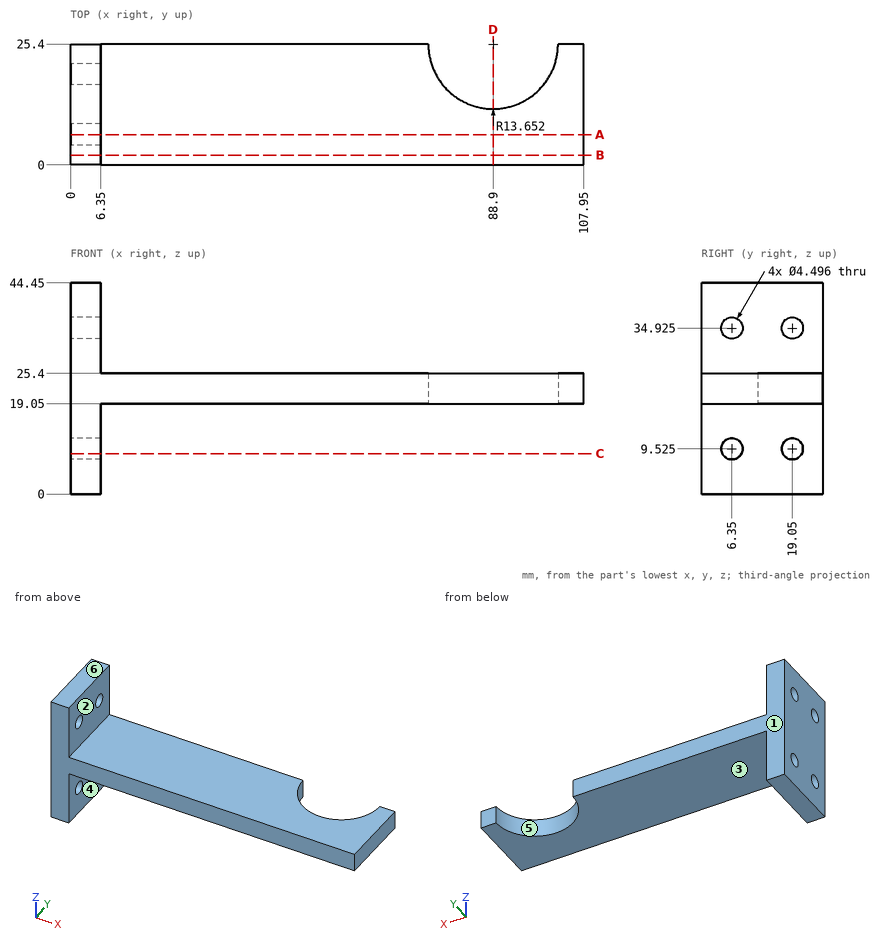
Answer from the drawing. Dimensions are ordinates in mm from the lowest x, y and z of the part. A direction names the side the tool comes from. Round coordinates to 2 decimals unless told otherwise and drop trailing zeros. Write each loop counter-clockwise with the first axis right and the second up, starting at its lowest first coordinate (ties: lowest second). Pieces come first, ordered by that corner, then holes.
1. Given pin 1 Ø10 at (y, z) = (7, 5.5) entering from +X; pin 2 Ø3.5 at (y, z) = (19.05, 34.925) entering from +X; pin 3 Ø7.5 at (x, y) = (35.5, 19) entering from -Z; pin 4 Ø1.5 at (x, y) = (28, 10.5) entering from +Z, each flat-ended and moving along its own axis, determine where each tip first touches the part or whether it passes through.
2. The part is cut by section B-B, the plane y = 2. Determine the outline of the cut face in (x, z).
3. Which of the six approach directions +Z, -Z, +X, -X, +Y, -Y give full straight-line access (tool end or side, diameter ignored) to the marked faces 1, 2 and 3?
4. The part is cut by section C-C, the plane z = 8.5. Determine the outline of the cut face in (x, y).
5. The part is cut by section A-A, the plane y = 6.35. Determine the outline of the cut face in (x, z).
6. Determine the mould class of the marked faces 4, 5 and 6 for opening direction X: pulls with the +X half, pulls with the -X half, needs draft (parallel to the pull), parting line crosses it, or undercut.
7. The part is cut by section D-D, the plane x = 88.9. Determine the outline of the cut face in (y, z).
8. Straight lines are drawn through the part: L1, parallel to Z at x = 2.5, y = 6.35; L2, parallel to Z at x = 18, y = 6.25; L3, parallel to X at y = 21, z = 39. For each, find the intervals that lie inside material, in ascending order.
Values:
1. pin 1: stops at x = 6.35
1. pin 2: passes through
1. pin 3: stops at z = 19.05
1. pin 4: stops at z = 25.4
2. outline: (0, 0) - (6.35, 0) - (6.35, 19.05) - (107.95, 19.05) - (107.95, 25.4) - (6.35, 25.4) - (6.35, 44.45) - (0, 44.45) - close
3. face 1: +Z, -Z, +X, -X, +Y
3. face 2: +Z, +X, +Y, -Y
3. face 3: -Z, +X, +Y, -Y
4. outline: (0, 0) - (6.35, 0) - (6.35, 4.35) - (0, 4.35) - close; (0, 8.35) - (6.35, 8.35) - (6.35, 17.05) - (0, 17.05) - close; (0, 21.05) - (6.35, 21.05) - (6.35, 25.4) - (0, 25.4) - close
5. outline: (0, 0) - (6.35, 0) - (6.35, 7.28) - (0, 7.28) - close; (0, 11.77) - (6.35, 11.77) - (6.35, 19.05) - (107.95, 19.05) - (107.95, 25.4) - (6.35, 25.4) - (6.35, 32.68) - (0, 32.68) - close; (0, 37.17) - (6.35, 37.17) - (6.35, 44.45) - (0, 44.45) - close
6. face 4: pulls with the +X half
6. face 5: undercut
6. face 6: needs draft
7. outline: (0, 19.05) - (11.75, 19.05) - (11.75, 25.4) - (0, 25.4) - close
8. L1: z = 0 to 7.28, 11.77 to 32.68, 37.17 to 44.45
8. L2: z = 19.05 to 25.4
8. L3: x = 0 to 6.35
